Design review of the part shown in the three views and the two pictorial views. Dimensions are in mm from the part's minimum x, y and z. Coordinates: 2 decimals unless noted, no trailing zeros. Write each loop counter-clockwise with the first axis right and the second up, starting at its lowest first coordinate (ties: lowest second). Pieces come first, ordered by that corner, then holes. Notation, with made-up numbers: (-3, -7) - (56, -7) arc R16 cw to (56, 18) - close; hole circle Ø4 at (79.5, 27.25). An arc over 180 degrees is marked (long way). Write each question's results on one line, items separated by ' | '.
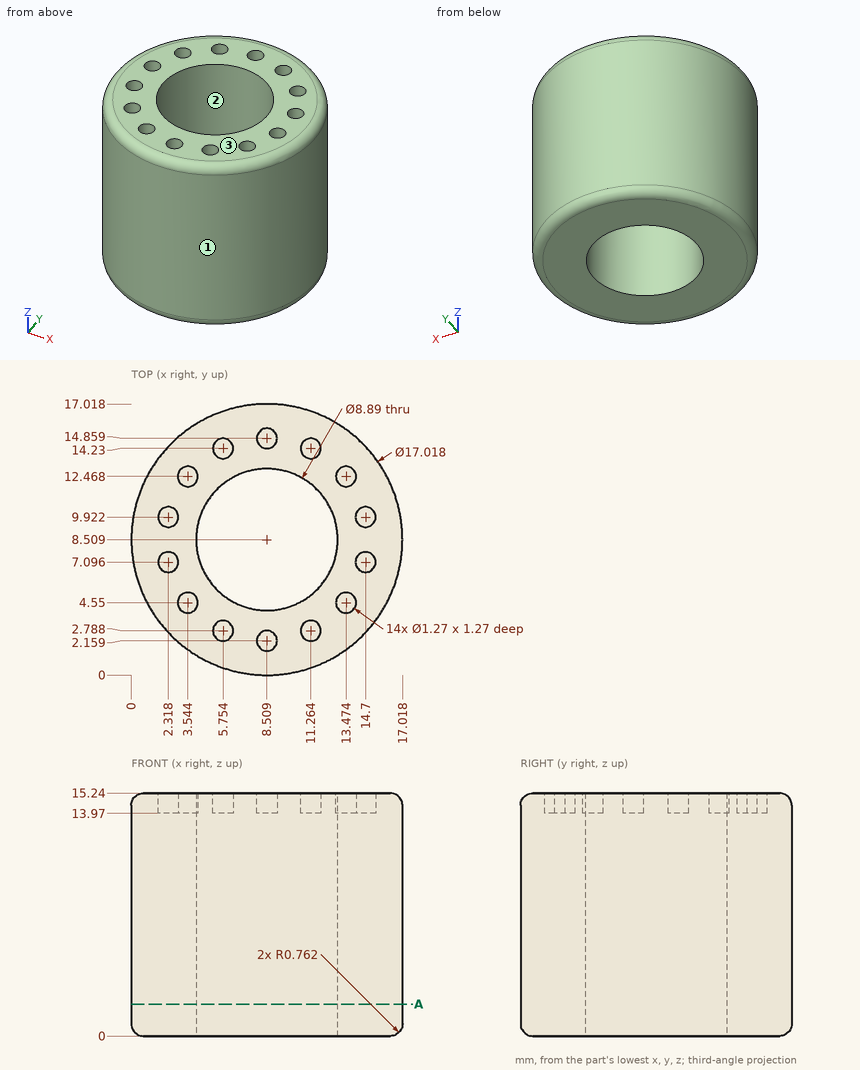
Q1. For pin 1 (1 mm diameter, centred on y = 11.5, z = 11, fed in from +X) (1 decimal); pin 2 (3 mm diameter, centred on x = 14, z = 12, fed in from -Y) (1 decimal), all flat-tipped, find the tip position at first contact; note any pin that passes through.
Results found:
pin 1: x = 16.6 | pin 2: y = 1
Q2. Wall thickness on line 1 along Y through (x, z) = (15, 14) (1 decimal); line 2 along X through (y, z) = (8.5, 9.75); line 3 along X through (y, z) = (6.75, 11) (1 decimal): over which ranges is each line inside the solid? List them lowest first. Write a range as from..to.
Results found:
line 1: 3..6.5, 7.7..9.4, 10.5..14 | line 2: 0..4.06, 12.95..17.02 | line 3: 0.2..4.4, 12.6..16.8
Q3. Take a section at A-A on z = 2. State the section outline as (x, y) points (1 decimal).
Results found:
outline: circle Ø17 at (8.5, 8.5); hole circle Ø8.9 at (8.5, 8.5)
Q4. Mouldability with a two-part tool opening along X and no side actions: class the marked faces 1, 2 and 3 as pulls with the +X half, pulls with the -X half, needs draft (parallel to the pull), parting line crosses it, or undercut.
Results found:
face 1: parting line crosses it | face 2: undercut | face 3: needs draft
